Read the model definition and answer for the solid it produces. Units are mm, in the model's axes. A direction names the side the tool comes from. Coordinates: 2 decimals unless noted, no trailing zeros. Order: outer loops, then holes, each group sorted by start corner. A loop starts at its lowest first (then second) coordinate and runs counter-clockwise, first axis right, second up. Notation, with made-up numbers: (9.5, 27.25) - (26.5, 27.25) arc R27 ccw to (26.5, 45.25) - close; hole circle Ø1 at (18, -40). An arc over 180 degrees is marked (long way). Answer as a JSON object with one key per item and string values. Group by question number.
Autodesk Inventor part; units mm, degrees
ref_plane "YZ Plane" through (0, 0, 0) normal (1, 0, 0) x (0, 1, 0)
ref_plane "XZ Plane" through (0, 0, 0) normal (0, 1, 0) x (-1, 0, 0)
ref_plane "XY Plane" through (0, 0, 0) normal (0, 0, 1) x (1, 0, 0)
sketch "Sketch2" plane through (0, 0, 0) normal (0, 1, 0) x (-1, 0, 0)
  line L0 (0, 0) -> (-37, 0)
  line L1 (-37, 0) -> (-37, -35)
  line L2 (-37, -35) -> (0, -35)
  line L3 (0, -35) -> (0, 0)
  dimension "d4" = 37
  dimension "d5" = 35
extrude "Extrusion2" add sketch "Sketch2" along normal blind 10
sketch "Sketch3" plane through (0, 10, 0) normal (0, 1, 0) x (1, 0, 0)
  point P0 (0, 0)
sketch "Sketch4" plane through (0, 10, 0) normal (0, 1, 0) x (1, 0, 0)
  line L0 (30.9066, 2.247) -> (16.0066, 2.247)
  line L1 (16.0066, 2.247) -> (16.0066, 7.247)
  line L2 (16.0066, 7.247) -> (15.0066, 7.247)
  line L3 (30.9066, 2.247) -> (30.9066, 9.047)
  line L4 (30.9066, 9.047) -> (35.2566, 9.047)
  line L5 (35.2566, 9.047) -> (35.2566, 11.047)
  line L6 (35.2566, 11.047) -> (30.9066, 11.047)
  line L7 (30.9066, 11.047) -> (30.9066, 31.847)
  line L8 (30.9066, 31.847) -> (8.3066, 31.847)
  line L9 (8.3066, 31.847) -> (8.3066, 11.047)
  line L10 (8.3066, 11.047) -> (3.9566, 11.047)
  line L11 (3.9566, 11.047) -> (3.9566, 9.047)
  line L12 (3.9566, 9.047) -> (8.3066, 9.047)
  line L13 (8.3066, 9.047) -> (8.3066, 8.147)
  line L14 (8.3066, 8.147) -> (15.0066, 7.247)
  point P0 (0, 0)
  dimension "d8" = 14.9
  dimension "d9" = 5
  dimension "d10" = 1
  dimension "d11" = 6.8
  dimension "d12" = 4.35
  dimension "d13" = 2
  dimension "d14" = 20.8
  dimension "d15" = 22.6
  dimension "d16" = 4.35
  dimension "d17" = 0.9
extrude "Extrusion3" cut sketch "Sketch4" against normal blind 5.85
chamfer "Chamfer1" distance 1 angle 45 4 edges at (37, 10, -17.5) (18.5, 10, -35) (0, 10, -17.5) (18.5, 10, 0)
properties part number "servo_sandbox"
1. A cutting plane is placed at A-A on y = 5. Write down the section's boundary in (x, z).
2. For a pull along Z with two mould halves and no side action, classify faces 3 (the flat face through (0, 4, -18)), 4 (the flat face through (35.257, 7, -10)), 5 (the flat face through (18.2, 9.5, -34.5)) as pulls with the +Z half, pulls with the -Z half, needs draft (parallel to the pull), parting line crosses it, or undercut.
3. Straight lines are drawn through the part: L1, parallel to Z at x = 33, y = 5.5; L2, parallel to X at y = 7.75, z = -5.5; L3, parallel to X at y = 8.75, z = -29. For each, find the intervals that lie inside material, in ascending order.
4. A cutting plane is placed at B-B on z = -13. Write down the section's boundary in (x, y).
5. For faces 1 (the flat face through (37, 4, -17)), 2 (the flat face through (15.5, 7.1, -7.247)), determine the directions among +Z, -Z, +X, -X, +Y, -Y from which every point of the face is accessible in a straight line to the end or side of a thin tool.
6. Given pin 1 (1.3 mm diameter, centred on x = 7, y = 8.5, fed in from +Z); pin 2 (12 mm diameter, centred on x = 14.5, z = -20, fed in from +Y), each flat-ended and moving along its own axis, determine where each tip first touches the part or whether it passes through.
7. A cutting plane is placed at C-C on x = 26. Write down the section's boundary in (y, z).
Derived:
{
 "1": {"outline": "(0, -35) - (37, -35) - (37, 0) - (0, 0) - close; hole (3.96, -11.05) - (8.31, -11.05) - (8.31, -31.85) - (30.91, -31.85) - (30.91, -11.05) - (35.26, -11.05) - (35.26, -9.05) - (30.91, -9.05) - (30.91, -2.25) - (16.01, -2.25) - (16.01, -7.25) - (15.01, -7.25) - (8.31, -8.15) - (8.31, -9.05) - (3.96, -9.05) - close"},
 "2": {"face 3": "needs draft", "face 4": "undercut", "face 5": "pulls with the -Z half"},
 "3": {"L1": "z = -35 to -11.05, -9.05 to 0", "L2": "x = 0 to 16.01, 30.91 to 37", "L3": "x = 0 to 8.31, 30.91 to 37"},
 "4": {"outline": "(0, 0) - (37, 0) - (37, 9) - (36, 10) - (30.91, 10) - (30.91, 4.15) - (8.31, 4.15) - (8.31, 10) - (1, 10) - (0, 9) - close"},
 "5": {"face 1": "+Z, -Z, +X, +Y, -Y", "face 2": "+Y"},
 "6": {"pin 1": "stops at z = 0", "pin 2": "stops at y = 4.15"},
 "7": {"outline": "(0, -35) - (9, -35) - (10, -34) - (10, -31.85) - (4.15, -31.85) - (4.15, -2.25) - (10, -2.25) - (10, -1) - (9, 0) - (0, 0) - close"}
}
